Part model, mm, in its own coordinate system. Face numbers are marked on the shaded views. A direction names the side the tool comes from. Coordinates: 2 decimals unless noted, no trailing zeros. Loops run counter-clockwise (first coordinate to the right, second up) from the corner with the lowest first, then second, coordinate; pieces in that order, holes last. Notation, with made-up numbers: M 63.25,49 L 121.25,49 A11 ccw 121.25,65 Z; hole C 0,-11.5 d6. An arc over 180 degrees is marked long. Answer as a JSON object with one key per item and string values. Group by question number.
1. 3-axis set-ups, long thin cutter, end or side, ignore diameter. For the marked faces 1 and 2: which of +Z, -Z, +X, -X, +Y, -Y reach the whole face in a straight line?
2. Saw through at A-A on y = 1.75. Count the separate pieces of the cut face and the enclosed holes in it, then the cut area to 3 significant figures.
3. Saw through at C-C on x = -25. Write the cut outline in (y, z), then the cut area to 3 significant figures.
4. Saw through at B-B on z = -25. Write the cut outline in (x, y), then the cut area to 3 significant figures.
5. Drill centre lines: L1, parallel to Z at x = -0.5, y = 1; L2, parallel to X at y = 3.25, z = 25; L3, parallel to X at y = 5.25, z = -25. Where is each one in solid material? Low to high.
6. Saw through at D-D on x = -6.5. Write the cut outline in (y, z).
7. Drop flat-ended pins along their axis: pin 1 Ø6 at (x, z) = (1.5, 27.5) entering from +Y; pin 2 Ø1 at (y, z) = (8, 45.5) entering from +X; pin 3 Ø2 at (y, z) = (10, 2) entering from -X; pin 4 Ø4 at (x, z) = (-25, 12.5) entering from -Y. Give the stop position or say it passes through.
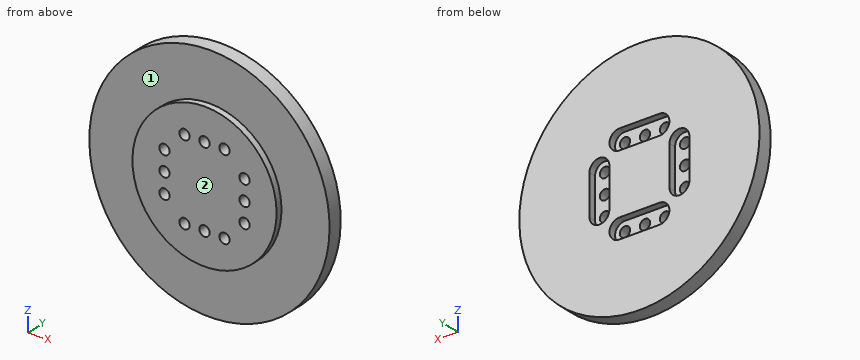
from build123d import *

# Parameters (mm, degrees)
SKETCH_1_R          = 45
EXTRUDE_1_DEPTH     = 4
SKETCH_2_R          = 75
EXTRUDE_2_DEPTH     = 9
SKETCH_3_R          = 3.2
CUT_EXTRUDE_1_DEPTH = 107.85972113
CUT_EXTRUDE_2_DEPTH = 4.5


with BuildPart() as part:
    # 草图1 → 凸台-拉伸1 (new body)
    with BuildSketch(Plane(origin=(0, 0, 0), x_dir=(1, 0, 0), z_dir=(0, 1, 0))):
        with Locations(Location((0, 0, 0), (0, 0, 270))):
            Circle(SKETCH_1_R)
    extrude(amount=EXTRUDE_1_DEPTH)

    # 草图2 → 凸台-拉伸2 (add)
    with BuildSketch(Plane(origin=(0, 4, 0), x_dir=(1, 0, 0), z_dir=(0, 1, 0))):
        with Locations(Location((0, 0, 0), (0, 0, 270))):
            Circle(SKETCH_2_R)
    extrude(amount=EXTRUDE_2_DEPTH)

    # 草图3 → 切除-拉伸1 (cut, through all)
    with BuildSketch(Plane(origin=(0, 13, 0), x_dir=(1, 0, 0), z_dir=(0, 1, 0))):
        with Locations(Location((-12.5, 25, 0), (0, 0, 270))):
            Circle(SKETCH_3_R)
        with Locations(Location((0, 25, 0), (0, 0, 270))):
            Circle(SKETCH_3_R)
        with Locations(Location((12.5, 25, 0), (0, 0, 270))):
            Circle(SKETCH_3_R)
        with Locations(Location((25, 0, 0), (0, 0, 270))):
            Circle(SKETCH_3_R)
        with Locations(Location((25, 12.5, 0), (0, 0, 270))):
            Circle(SKETCH_3_R)
        with Locations(Location((25, -12.5, 0), (0, 0, 270))):
            Circle(SKETCH_3_R)
    cut_extrude_1 = extrude(amount=-CUT_EXTRUDE_1_DEPTH, mode=Mode.SUBTRACT)

    # 镜向1: 切除-拉伸1 across plane
    add(cut_extrude_1.mirror(Plane(origin=(0, 0, 0), x_dir=(0, 0, 1), z_dir=(1, 0, 0))), mode=Mode.SUBTRACT)

    # 镜向1 at the second plane: 切除-拉伸1 across plane
    add(cut_extrude_1.mirror(Plane.XY), mode=Mode.SUBTRACT)

    # 草图4 → 切除-拉伸2 (cut)
    with BuildSketch(Plane(origin=(0, 13, 0), x_dir=(1, 0, 0), z_dir=(0, 1, 0))):
        with BuildLine():
            Line((-12.5, 31.2), (12.5, 31.2))
            ThreePointArc((12.5, 31.2), (18.7, 25), (12.5, 18.8))
            Line((12.5, 18.8), (-12.5, 18.8))
            ThreePointArc((-12.5, 18.8), (-18.7, 25), (-12.5, 31.2))
        make_face()
        with BuildLine():
            Line((-18.8, 12.5), (-18.8, -12.5))
            ThreePointArc((-18.8, -12.5), (-25, -18.7), (-31.2, -12.5))
            Line((-31.2, -12.5), (-31.2, 12.5))
            ThreePointArc((-31.2, 12.5), (-25, 18.7), (-18.8, 12.5))
        make_face()
    cut_extrude_2 = extrude(amount=-CUT_EXTRUDE_2_DEPTH, mode=Mode.SUBTRACT)

    # 镜向2: 切除-拉伸2 across plane
    add(cut_extrude_2.mirror(Plane(origin=(0, 0, 0), x_dir=(0, 0, 1), z_dir=(1, 0, 0))), mode=Mode.SUBTRACT)

    # 镜向2 at the second plane: 切除-拉伸2 across plane
    add(cut_extrude_2.mirror(Plane.XY), mode=Mode.SUBTRACT)


solid = part.part
Outcome:
{
 "1": {"face 1": "-Y", "face 2": "+Z, -Z, +X, -X, -Y"},
 "2": {"separate pieces": "1", "enclosed holes": "12", "area": "5,980 mm²"},
 "3": {"outline": "M 0,-37.42 L 4,-37.42 L 4,-70.71 L 13,-70.71 L 13,-18.7 L 8.5,-18.7 L 8.5,-15.7 L 0,-15.7 Z; M 0,-9.3 L 8.5,-9.3 L 8.5,-3.2 L 0,-3.2 Z; M 0,3.2 L 8.5,3.2 L 8.5,9.3 L 0,9.3 Z; M 0,15.7 L 8.5,15.7 L 8.5,18.7 L 13,18.7 L 13,70.71 L 4,70.71 L 4,37.42 L 0,37.42 Z", "area": "1,240 mm²"},
 "4": {"outline": "M -70.71,4 L -37.42,4 L -37.42,0 L -15.7,0 L -15.7,8.5 L -18.7,8.5 L -18.7,13 L -70.71,13 Z; M -9.3,0 L -3.2,0 L -3.2,8.5 L -9.3,8.5 Z; M 3.2,0 L 9.3,0 L 9.3,8.5 L 3.2,8.5 Z; M 15.7,0 L 37.42,0 L 37.42,4 L 70.71,4 L 70.71,13 L 18.7,13 L 18.7,8.5 L 15.7,8.5 Z", "area": "1,240 mm²"},
 "5": {"L1": "z = -45 to -28.16, -21.84 to 21.84, 28.16 to 45", "L2": "x = -37.42 to -15.7, -9.3 to -3.2, 3.2 to 9.3, 15.7 to 37.42", "L3": "x = -70.71 to -15.7, -9.3 to -3.2, 3.2 to 9.3, 15.7 to 70.71"},
 "6": {"outline": "M 0,-44.53 L 4,-44.53 L 4,-74.72 L 13,-74.72 L 13,-31.2 L 8.5,-31.2 L 8.5,-18.8 L 13,-18.8 L 13,18.8 L 8.5,18.8 L 8.5,31.2 L 13,31.2 L 13,74.72 L 4,74.72 L 4,44.53 L 0,44.53 Z"},
 "7": {"pin 1": "stops at y = 8.5", "pin 2": "stops at x = 60", "pin 3": "stops at x = -74.99", "pin 4": "passes through"}
}
